Read the model definition and answer for the solid it produces. Units are mm, in the model's axes. Face numbers are marked on the shaded views. A direction names the side the tool comes from. Coordinates: 2 decimals unless noted, no trailing zeros. Loops run counter-clockwise (first coordinate to the right, second up) from the corner with the lowest first, then second, coordinate; pieces in that order, holes last.
Q1. Section B-B (x = -1) is taken. Give the vertices of the cut face in (y, z), then the cut area to 3 significant figures.
Q2. Section A-A (y = 24.5) is taken. Give the vertices of the cut face in (x, z), then the cut area to 3 significant figures.
Q3. The mould has two halves that part along Z. Classify the marked faces 1, 2, 3 and 4: pulls with the +Z half, pulls with the -Z half, needs draft (parallel to the pull), parting line crosses it, or undercut.
Q4. Flat-ended cylindrical pins translate along their axes: P1, Ø14, axis at y = 16, z = 14, coming from the -X side; P2, Ø5, axis at x = 36.5, y = 22.5, coming from the -Z side; P3, Ø2, axis at x = 20.5, z = -17.5, coming from the +Y side; P4, Ø2, axis at x = -10.65, y = 20.03, coming from the -Z side. Find the tip coordinate at first contact, or state that the pin passes through.
Q5. Section C-C (z = -10) is taken. Give the vertices of the cut face in (x, y), then the cut area to 3 significant figures.
Q6. Section D-D (y = 11) is taken. Give the vertices of the cut face in (x, z).
Q7. Straight lines are drawn through the part: line 1 (X direction, y = 30.03, z = 16.25); line 2 (Z direction, x = -1, y = 11.5); line 3 (Y direction, x = 3, z = 17). For each, find the intervals that lie inside material, in ascending order.
Q8. Which of the six approach directions +Z, -Z, +X, -X, +Y, -Y give full straight-line access (tool end or side, diameter ignored) to the marked faces 5, 6 and 7?
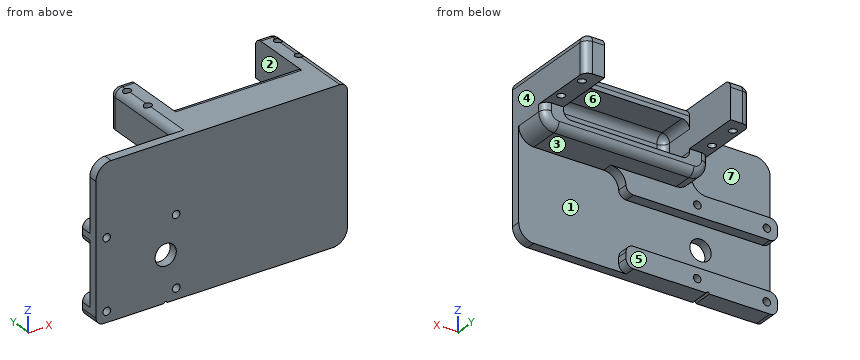
from build123d import *

# Parameters (mm, degrees)
SKETCH1_W             = 83
SKETCH1_H             = 50
BOSS_EXTRUDE1_DEPTH   = 3
SKETCH2_W             = 50
SKETCH2_H             = 7
BOSS_EXTRUDE2_DEPTH   = 3.5
SKETCH3_W             = 6.457447236
SKETCH3_H             = 12.6
BOSS_EXTRUDE3_DEPTH   = 31.93
M3X0_5_TAPPED_HOLE1_D = 2.5
SKETCH6_W             = 54.514894472
SKETCH6_H             = 20
BOSS_EXTRUDE4_DEPTH   = 12.13
SKETCH10_W            = 41.6
SKETCH10_H            = 12
CUT_EXTRUDE2_DEPTH    = 12.13
FILLET1_R             = 5
FILLET2_R             = 5
FILLET3_R             = 2.5
FILLET4_R             = 2.5
FILLET5_R             = 2.5
M3X0_5_TAPPED_HOLE2_D = 2.5
SKETCH9_R             = 3.5
CUT_EXTRUDE1_DEPTH    = 59.023916735
FILLET6_R             = 2.5
CUT_EXTRUDE3_DEPTH    = 60.727338073


with BuildPart() as part:
    # Sketch1 → Boss-Extrude1 (new body)
    with BuildSketch(Plane(origin=(0, 0, 0), x_dir=(1, 0, 0), z_dir=(0, 1, 0))):
        Rectangle(SKETCH1_W, SKETCH1_H)
    extrude(amount=BOSS_EXTRUDE1_DEPTH)

    # Sketch2 → Boss-Extrude2 (add)
    with BuildSketch(Plane(origin=(0, 3, 0), x_dir=(1, 0, 0), z_dir=(0, 1, 0))):
        with Locations((-16.5, 21.5)):
            Rectangle(SKETCH2_W, SKETCH2_H)
        with Locations((-16.5, -1.5)):
            Rectangle(SKETCH2_W, SKETCH2_H)
    extrude(amount=BOSS_EXTRUDE2_DEPTH)

    # Sketch3 → Boss-Extrude3 (add)
    with BuildSketch(Plane(origin=(0, 3, 0), x_dir=(1, 0, 0), z_dir=(0, 1, 0))):
        with Locations((38.271276382, -18.7)):
            Rectangle(SKETCH3_W, SKETCH3_H)
        with Locations((-9.786170854, -18.7)):
            Rectangle(SKETCH3_W, SKETCH3_H)
    extrude(amount=BOSS_EXTRUDE3_DEPTH)

    # M3x0.5 Tapped Hole1 (through all)
    with Locations(Plane(origin=(0, 0, 12.4), x_dir=(-1, 0, 0), z_dir=(0, 0, -1))):
        with Locations((-39.132166065, 30.03), (-39.132166065, 20.03), (10.647060537, 20.03), (10.647060537, 30.03)):
            Hole(M3X0_5_TAPPED_HOLE1_D / 2)

    # Sketch6 → Boss-Extrude4 (add)
    with BuildSketch(Plane(origin=(0, 3, 0), x_dir=(1, 0, 0), z_dir=(0, 1, 0))):
        with Locations((14.242552764, -15)):
            Rectangle(SKETCH6_W, SKETCH6_H)
    extrude(amount=BOSS_EXTRUDE4_DEPTH)

    # Sketch10 → Cut-Extrude2 (cut)
    with BuildSketch(Plane(origin=(0, 15.13, 0), x_dir=(1, 0, 0), z_dir=(0, 1, 0))):
        with Locations((14.242552764, -15)):
            Rectangle(SKETCH10_W, SKETCH10_H)
    extrude(amount=-CUT_EXTRUDE2_DEPTH, mode=Mode.SUBTRACT)

    # Fillet1
    fillet1_edges = [part.edges().sort_by_distance(p)[0] for p in [
        (8.5, 4.75, 5),
        (41.5, 9.065, 5),
        (-13.014894472, 4.75, 5),
    ]]
    fillet(fillet1_edges, radius=FILLET1_R)

    # Fillet2
    fillet2_edges = [part.edges().sort_by_distance(p)[0] for p in [
        (-13.014894472, 10.815, 5),
        (-41.5, 1.5, 25),
        (41.5, 1.5, -25),
    ]]
    fillet(fillet2_edges, radius=FILLET2_R)

    # Fillet3
    fillet3_edges = [part.edges().sort_by_distance(p)[0] for p in [
        (8.5, 4.75, -18),
        (-41.5, 4.75, -18),
        (-41.5, 4.75, -2),
        (8.5, 4.75, -2),
        (8.5, 4.75, -25),
        (-41.5, 4.75, 5),
        (-41.5, 3.25, -25),
    ]]
    fillet(fillet3_edges, radius=FILLET3_R)

    # Fillet4
    fillet4_edges = [part.edges().sort_by_distance(p)[0] for p in [
        (14.242552764, 15.13, 5),
        (40.035533906, 15.13, 6.464466094),
        (-13.014894472, 15.13, 11.2),
        (-11.550428378, 15.13, 6.464466094),
        (41.5, 15.13, 11.2),
        (14.242552764, 15.13, 25),
    ]]
    fillet(fillet4_edges, radius=FILLET4_R)

    # Fillet5
    # the kernel refuses this fillet: 2.5 mm, written as the material it takes off along each edge
    with BuildSketch(Plane(origin=(39, 32.43, 22.5), x_dir=(1, 0, 0), z_dir=(0, 0, 1))) as fillet5_piece_1_section:
        Polygon((0, 0), (FILLET5_R * 1.02, 0), (FILLET5_R * 1.02, FILLET5_R * 1.02), (0, FILLET5_R * 1.02), align=None)
    fillet5_piece_1 = extrude(amount=FILLET5_R * 1.02, mode=Mode.PRIVATE)
    fillet5_piece_1 = fillet5_piece_1 - Plane(origin=(39, 32.43, 22.5), x_dir=(-0.7071067811865475, -0.7071067811865475, 0), z_dir=(0, 0, 1)) * Sphere(FILLET5_R, mode=Mode.PRIVATE)
    add(fillet5_piece_1, mode=Mode.SUBTRACT)
    with BuildSketch(Plane(origin=(-10.514894472, 32.43, 22.5), x_dir=(-1, 0, 0), z_dir=(0, 0, 1))) as fillet5_piece_2_section:
        Polygon((0, 0), (FILLET5_R * 1.02, 0), (FILLET5_R * 1.02, -FILLET5_R * 1.02), (0, -FILLET5_R * 1.02), align=None)
    fillet5_piece_2 = extrude(amount=FILLET5_R * 1.02, mode=Mode.PRIVATE)
    fillet5_piece_2 = fillet5_piece_2 - Plane(origin=(-10.514894472, 32.43, 22.5), x_dir=(0.7071067811865475, -0.7071067811865475, 0), z_dir=(0, 0, 1)) * Sphere(FILLET5_R, mode=Mode.PRIVATE)
    add(fillet5_piece_2, mode=Mode.SUBTRACT)
    with BuildSketch(Plane(origin=(39, 34.93, 25), x_dir=(0, -1, 0), z_dir=(-1, 0, 0))) as fillet5_piece_3:
        with BuildLine():
            CenterArc((FILLET5_R, -FILLET5_R), FILLET5_R, 90, 90)
            Line((0, -FILLET5_R), (0, 0))
            Line((0, 0), (FILLET5_R, 0))
        make_face()
    extrude(amount=10.207447236, mode=Mode.SUBTRACT)
    with BuildSketch(Plane(origin=(41.5, 34.93, 6.15), x_dir=(-1, 0, 0), z_dir=(0, 0, 1)), Plane(origin=(-13.014894472, 34.93, 6.15), x_dir=(0, -1, 0), z_dir=(0, 0, 1))) as fillet5_piece_4:
        with BuildLine():
            CenterArc((FILLET5_R, FILLET5_R), FILLET5_R, 180, 90)
            Line((0, FILLET5_R), (0, 0))
            Line((0, 0), (FILLET5_R, 0))
        make_face()
    extrude(amount=16.35, mode=Mode.SUBTRACT)
    with BuildSketch(Plane(origin=(-10.514894472, 34.93, 25), x_dir=(0, -1, 0), z_dir=(1, 0, 0))) as fillet5_piece_5:
        with BuildLine():
            CenterArc((FILLET5_R, FILLET5_R), FILLET5_R, 180, 90)
            Line((0, FILLET5_R), (0, 0))
            Line((0, 0), (FILLET5_R, 0))
        make_face()
    extrude(amount=10.207447236, mode=Mode.SUBTRACT)
    with BuildSketch(Plane(origin=(-13.014894472, 32.43, 25), x_dir=(1, 0, 0), z_dir=(0, -1, 0))) as fillet5_piece_6:
        with BuildLine():
            CenterArc((FILLET5_R, -FILLET5_R), FILLET5_R, 90, 90)
            Line((0, -FILLET5_R), (0, 0))
            Line((0, 0), (FILLET5_R, 0))
        make_face()
    extrude(amount=29.43, mode=Mode.SUBTRACT)
    with BuildSketch(Plane(origin=(41.5, 32.43, 25), x_dir=(-1, 0, 0), z_dir=(0, -1, 0))) as fillet5_piece_7:
        with BuildLine():
            CenterArc((FILLET5_R, FILLET5_R), FILLET5_R, 180, 90)
            Line((0, FILLET5_R), (0, 0))
            Line((0, 0), (FILLET5_R, 0))
        make_face()
    extrude(amount=38.68, mode=Mode.SUBTRACT)

    # M3x0.5 Tapped Hole2 (through all)
    with Locations(Plane(origin=(0, 6.5, 0), x_dir=(1, 0, 0), z_dir=(0, 1, 0))):
        with Locations((-37.99546971, -1.433732), (-15.066268, -1.49546971), (-15.00453029, 21.433732), (-37.933732, 21.49546971)):
            Hole(M3X0_5_TAPPED_HOLE2_D / 2)

    # Sketch9 → Cut-Extrude1 (cut, through all)
    with BuildSketch(Plane(origin=(0, 3, 0), x_dir=(1, 0, 0), z_dir=(0, 1, 0))):
        with Locations(Location((-18.5, 10, 0), (0, 0, 270))):
            Circle(SKETCH9_R)
    extrude(amount=-CUT_EXTRUDE1_DEPTH, mode=Mode.SUBTRACT)

    # Fillet6
    fillet6_edges = [part.edges().sort_by_distance(p)[0] for p in [
        (-6.557447236, 9.065, 21),
        (-6.557447236, 9.065, 9),
        (35.042552764, 9.065, 9),
        (35.042552764, 9.065, 21),
        (-6.557447236, 3, 15),
        (14.242552764, 3, 9),
        (35.042552764, 3, 15),
        (14.242552764, 3, 21),
    ]]
    fillet(fillet6_edges, radius=FILLET6_R)

    # Sketch11 → Cut-Extrude3 (cut, through all)
    with BuildSketch(Plane.XZ):
        with BuildLine():
            Line((-19, -25), (-18, -25))
            ThreePointArc((-18, -25), (-18.5, -24.5), (-19, -25))
        make_face()
    extrude(amount=-CUT_EXTRUDE3_DEPTH, mode=Mode.SUBTRACT)


solid = part.part
Numbers:
1. outline: (0, -25) - (6.5, -25) - (6.5, -18) - (3, -18) - (3, -2) - (6.5, -2) - (6.5, 5) - (12.63, 5) arc R2.5 ccw to (15.13, 7.5) - (15.13, 9) - (5.5, 9) arc R2.5 cw to (3, 11.5) - (3, 18.5) arc R2.5 cw to (5.5, 21) - (15.13, 21) - (15.13, 22.5) arc R2.5 ccw to (12.63, 25) - (0, 25) - close
1. area: 296 mm2
2. outline: (-13.01, 12.4) - (-6.56, 12.4) - (-6.56, 25) - (-10.51, 25) arc R2.5 ccw to (-13.01, 22.5) - close; (35.04, 12.4) - (41.5, 12.4) - (41.5, 22.5) arc R2.5 ccw to (39, 25) - (35.04, 25) - close
2. area: 160 mm2
3. face 1: undercut
3. face 2: undercut
3. face 3: pulls with the -Z half
3. face 4: needs draft
4. P1: stops at x = -13.01
4. P2: stops at z = 12.4
4. P3: stops at y = 3
4. P4: passes through
5. outline: (-41.5, 0) - (-22, 0) - (-22, 3) - (-41.5, 3) - close; (-15, 0) - (41.5, 0) - (41.5, 3) - (-15, 3) - close
5. area: 228 mm2
6. outline: (-13.01, 10) arc R5 ccw to (-8.01, 5) - (36.5, 5) arc R5 ccw to (41.5, 10) - (41.5, 22.5) arc R2.5 ccw to (39, 25) - (-10.51, 25) arc R2.5 ccw to (-13.01, 22.5) - close; hole (-6.56, 11.5) arc R2.5 ccw to (-4.06, 9) - (32.54, 9) arc R2.5 ccw to (35.04, 11.5) - (35.04, 18.5) arc R2.5 ccw to (32.54, 21) - (-4.06, 21) arc R2.5 ccw to (-6.56, 18.5) - close
7. line 1: x = -13.01 to -11.9, -9.4 to -6.56, 35.04 to 37.88, 40.38 to 41.5
7. line 2: z = 5 to 9, 21 to 25
7. line 3: y = 0 to 3
8. face 5: -Z, +X, -X, +Y
8. face 6: +Y
8. face 7: +Z, -X, +Y
